Geometry check sheet. Reference: the model listing, model coordinates, mm. A direction names the side the tool comes from. Coordinates: 2 decimals unless noted, no trailing zeros. Write each loop counter-clockwise with the first axis right and the second up, starting at its lowest first coordinate (ties: lowest second). Pieces come first, ordered by that corner, then holes.
from build123d import *

# Parameters (mm, degrees)
SKETCH_1_R          = 20
EXTRUDE_1_DEPTH     = 20
CUT_EXTRUDE_1_DEPTH = 22.5
SKETCH_3_R          = 1.62
SKETCH_3_R_2        = 1.5
CUT_EXTRUDE_2_DEPTH = 22.5


with BuildPart() as part:
    # 草图1 → 凸台-拉伸1 (new body)
    with BuildSketch(Plane.XY):
        Circle(SKETCH_1_R)
    extrude(amount=EXTRUDE_1_DEPTH)

    # 草图2 → 切除-拉伸1 (cut)
    with BuildSketch(Plane.XY.offset(20)):
        with BuildLine():
            Line((4.769696007, -1.5), (3.2, -1.5))
            Line((3.2, -1.5), (3.2, 1.5))
            Line((3.2, 1.5), (4.769696007, 1.5))
            ThreePointArc((4.769696007, 1.5), (-5, 0), (4.769696007, -1.5))
        make_face()
    extrude(amount=-CUT_EXTRUDE_1_DEPTH, mode=Mode.SUBTRACT)

    # 草图3 → 切除-拉伸2 (cut)
    with BuildSketch(Plane.XY.offset(20)):
        with Locations((11, 7.5)):
            Circle(SKETCH_3_R)
        with Locations((-11, -7.5)):
            Circle(SKETCH_3_R)
        with Locations((11, -6.5)):
            Circle(SKETCH_3_R_2)
    extrude(amount=-CUT_EXTRUDE_2_DEPTH, mode=Mode.SUBTRACT)


solid = part.part
1. Gauge pin test, flat ends, axial feed: pin 1 Ø4 at (x, z) = (-11, 16) entering from -Y; pin 2 Ø4 at (y, z) = (7, 16.5) entering from +X; pin 3 Ø1.7 at (x, z) = (4.5, 13) entering from +Y. Record the tip position at first contact, or that the pin passes through.
Computed values:
pin 1: stops at y = -17.86
pin 2: stops at x = 19.36
pin 3: stops at y = 19.66
2. Access from +Z, -Z, +X, -X, +Y, -Y to the whole of each face (thin tool, end or side, straight path). Record for faces 4 (the flat face through (4, 1.5, 10)), 5 (the flat face through (4, 0, 0)).
Computed values:
face 4: +Z, -Z
face 5: -Z, +X, -X, +Y, -Y
3. Sectioned sample at A-A, the plane y = 0. Record the boundary of the cut face in (x, z).
Computed values:
outline: (-20, 0) - (-5, 0) - (-5, 20) - (-20, 20) - close; (3.2, 0) - (20, 0) - (20, 20) - (3.2, 20) - close
4. Sectioned sample at C-C, the plane x = 11. Record the boundary of the cut face in (y, z).
Computed values:
outline: (-16.7, 0) - (-8, 0) - (-8, 20) - (-16.7, 20) - close; (-5, 0) - (5.88, 0) - (5.88, 20) - (-5, 20) - close; (9.12, 0) - (16.7, 0) - (16.7, 20) - (9.12, 20) - close
5. Draft check along X on faces 1 (the flat face through (4, 0, 20)), 2 (the cylindrical face through (-4.336, -19.524, 9.86)), 3 (the cylindrical face through (12.496, 6.88, 10.14)). Enter one of: released by +X, released by -X, zero draft, split by the parting line, or undercut.
Computed values:
face 1: zero draft
face 2: split by the parting line
face 3: undercut
6. Sectioned sample at B-B, the plane z = 7. Record the boundary of the cut face in (x, y).
Computed values:
outline: circle Ø40 at (0, 0); hole circle Ø3.24 at (-11, -7.5); hole (3.2, -1.5) - (3.2, 1.5) - (4.77, 1.5) arc R5 ccw (long way) to (4.77, -1.5) - close; hole circle Ø3.24 at (11, 7.5); hole circle Ø3 at (11, -6.5)
7. Sectioned sample at D-D, the plane x = -11. Record the boundary of the cut face in (y, z), and give its area (3 significant figures).
Computed values:
outline: (-16.7, 0) - (-9.12, 0) - (-9.12, 20) - (-16.7, 20) - close; (-5.88, 0) - (16.7, 0) - (16.7, 20) - (-5.88, 20) - close
area: 603 mm2
8. Thickness scan on line 1 along Y through (x, z) = (0, 9.5); line 2 along Y through (x, z) = (3, 9); line 3 along Y through (x, z) = (11, 4.75). Record the ranges inside material, lowest first.
Computed values:
line 1: y = -20 to -5, 5 to 20
line 2: y = -19.77 to -4, 4 to 19.77
line 3: y = -16.7 to -8, -5 to 5.88, 9.12 to 16.7
